Check sheet for the drawn part. Datum: minimum x, y, z corner. Units: mm. A direction names the side the tool comes from. Coordinates: 2 decimals unless noted, no trailing zeros. Write each loop counter-clockwise with the first axis right and the second up, starting at its lowest first coordinate (ties: lowest second). Pieces come first, ordered by that corner, then holes. Notation, with made-up numbers: (2.5, 34) -> (51.5, 34) arc R19 ccw to (51.5, 40) -> close; hole circle Ø7 at (-9.75, -7.75). An arc over 180 degrees is marked (long way). Answer in a Markdown table with one row per item.
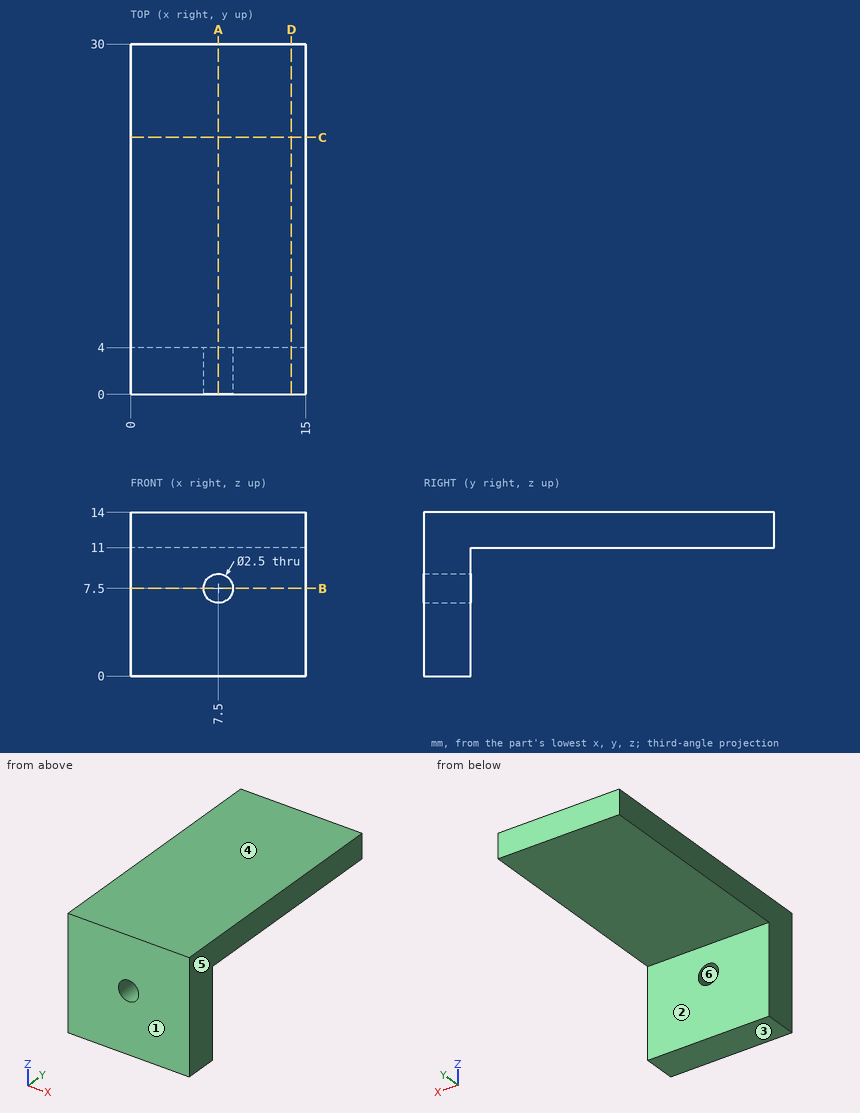
1. Release check for a two-part mould opening along Z. For the marked faces 3, 4, 5 and 6 record: released by +Z, released by -Z, zero draft, split by the parting line, or undercut.
Findings below:
| item | result |
|---|---|
| face 3 | released by -Z |
| face 4 | released by +Z |
| face 5 | zero draft |
| face 6 | undercut |
2. Access from +Z, -Z, +X, -X, +Y, -Y to the whole of each face (thin tool, end or side, straight path). Record for the marked faces 1 and 2.
Findings below:
| item | result |
|---|---|
| face 1 | +Z, -Z, +X, -X, -Y |
| face 2 | -Z, +X, -X, +Y |
3. Sectioned sample at D-D, the plane x = 13.75. Record the cut outline in (y, z).
Findings below:
| item | result |
|---|---|
| outline | (0, 0) -> (4, 0) -> (4, 11) -> (30, 11) -> (30, 14) -> (0, 14) -> close |
4. Sectioned sample at C-C, the plane y = 22. Record the cut outline in (x, z), and give its area (3 significant figures).
Findings below:
| item | result |
|---|---|
| outline | (0, 11) -> (15, 11) -> (15, 14) -> (0, 14) -> close |
| area | 45.0 mm² |
5. Go/stop test with flat-tipped pins: pin 1 (4 mm diameter, centred on y = 12.5, z = 10, fed in from +X); pin 2 (5.5 mm diameter, centred on x = 9, z = 8, fed in from +Y); pin 3 (7.5 mm diameter, centred on x = 8.5, y = 11.5, fed in from -Z); pin 4 (1.5 mm diameter, centred on x = 7.5, z = 7.5, fed in from -Y). Record where each tip stops, or that it passes through.
Findings below:
| item | result |
|---|---|
| pin 1 | stops at x = 15 |
| pin 2 | stops at y = 4 |
| pin 3 | stops at z = 11 |
| pin 4 | passes through |
6. Sectioned sample at B-B, the plane z = 7.5. Record the cut outline in (x, y).
Findings below:
| item | result |
|---|---|
| outline | (0, 0) -> (6.25, 0) -> (6.25, 4) -> (0, 4) -> close; (8.75, 0) -> (15, 0) -> (15, 4) -> (8.75, 4) -> close |
7. Sectioned sample at A-A, the plane x = 7.5. Record the cut outline in (y, z).
Findings below:
| item | result |
|---|---|
| outline | (0, 0) -> (4, 0) -> (4, 6.25) -> (0, 6.25) -> close; (0, 8.75) -> (4, 8.75) -> (4, 11) -> (30, 11) -> (30, 14) -> (0, 14) -> close |
8. Material ranges on probe 1 along Z at (x, y) = (7.5, 1.2); probe 2 along Y at (x, z) = (7.25, 4.5); probe 3 along X at (y, z) = (1.35, 7.5), recorded low to high. Write a range as from..to.
Findings below:
| item | result |
|---|---|
| probe 1 | z = 0..6.25, 8.75..14 |
| probe 2 | y = 0..4 |
| probe 3 | x = 0..6.25, 8.75..15 |
